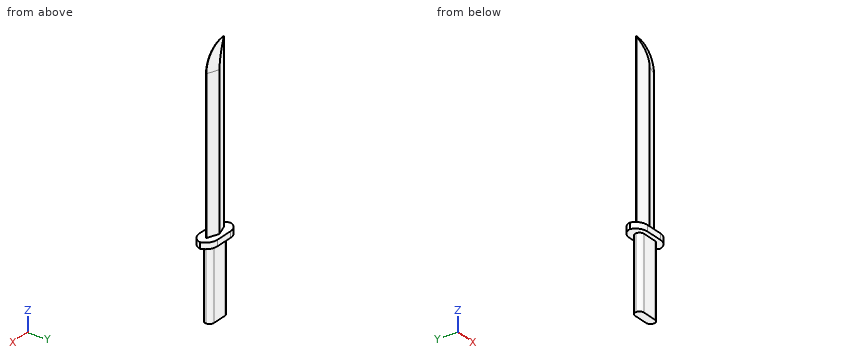
from build123d import *

# Parameters (mm, degrees)
F1_DEPTH     = 19.05
F2_W         = 88.9
F2_H         = 38.1
F3_DEPTH     = 12.7
F4_W         = 50.8
F4_H         = 381
F5_DEPTH     = 19.05
F6_R         = 50.79999
F7_T1_DEPTH  = 434.1925462068
F7_T3_DEPTH  = 317.50001
F7_T5_DEPTH  = 65.8925562068
F7_T8_ANGLE  = 90
F7_T10_ANGLE = 90
F8_R         = 9.52499
F9_T1_DEPTH  = 139.7


# Not quite as in the source:
# - a fillet or chamfer that OpenCascade refuses, or shapes differently, is made with other operations: its cross-section is extruded or revolved along the edge and cut away or added
# - a fillet or chamfer is up to 0.001 mm smaller than in the source, because OpenCascade refuses the exact size


with BuildPart() as f1:
    # F0 (on Front) → F1 (new body)
    with BuildSketch(Plane.XZ):
        Polygon((-25.4, -86.237093463), (0, -86.237093463), (25.4, -86.237093463), (25.4, 66.162906537), (-25.4, 66.162906537), align=None)
    extrude(amount=F1_DEPTH)

    # F2 (on face) → F3 (join)
    with BuildSketch(Plane.XY.offset(66.162906537)):
        with Locations((0, -9.525)):
            Rectangle(F2_W, F2_H)
    extrude(amount=F3_DEPTH)

    # F4 (on face) → F5 (join)
    with BuildSketch(Plane(origin=(0, 0, 0), x_dir=(-1, 0, 0), z_dir=(0, 1, 0))):
        with Locations((0, 256.662906537)):
            Rectangle(F4_W, F4_H)
    extrude(amount=-F5_DEPTH)

    # F6 (radius 50.8 in the source; OpenCascade refuses exactly that, so slightly less here)
    f6_edges = [f1.edges().sort_by_distance(p)[0] for p in [
        (25.4, -9.525, 447.162907),
    ]]
    fillet(f6_edges, radius=F6_R)

    # F7: chamfer of 25.4 x 9.2448439504 on 6 edges, made by hand

    # F7_s2 → F7_t1 (cut)
    with BuildSketch(Plane.XY.offset(78.862906537)):
        Polygon((0, 0), (-25.4, -9.2448439504), (-25.4, 0), align=None)
        Polygon((0, -19.05), (-25.4, -9.8051560496), (-25.4, -19.05), align=None)
    extrude(amount=F7_T1_DEPTH, mode=Mode.SUBTRACT)

    # F7_s4 → F7_t3 (cut)
    with BuildSketch(Plane.XY.offset(78.862906537)):
        Polygon((25.4, -9.2448439504), (0, 0), (25.4, 0), align=None)
        Polygon((25.4, -9.8051560496), (0, -19.05), (25.4, -19.05), align=None)
    extrude(amount=F7_T3_DEPTH, mode=Mode.SUBTRACT)

    # F7_s6 → F7_t5 (cut)
    with BuildSketch(Plane.YZ.offset(-91.2925462068)):
        Polygon((-19.05, 421.762906537), (-9.8051560496, 447.162906537), (-19.05, 447.162906537), align=None)
        Polygon((0, 421.762906537), (-9.2448439504, 447.162906537), (0, 447.162906537), align=None)
    extrude(amount=F7_T5_DEPTH, mode=Mode.SUBTRACT)

    # F7_s7 → F7_t8 (revolve, cut)
    with BuildSketch(Plane.XY.offset(396.362916537)):
        Polygon((0, 0), (25.4, -9.2448439504), (25.4, 0), align=None)
    revolve(axis=Axis((-25.39999, 0, 396.362916537), (0, -1, 0)), revolution_arc=F7_T8_ANGLE, mode=Mode.SUBTRACT)

    # F7_s9 → F7_t10 (revolve, cut)
    with BuildSketch(Plane.XY.offset(396.362916537)):
        Polygon((25.4, -9.8051560496), (0, -19.05), (25.4, -19.05), align=None)
    revolve(axis=Axis((-25.39999, -19.05, 396.362916537), (0, -1, 0)), revolution_arc=F7_T10_ANGLE, mode=Mode.SUBTRACT)

    # F8 (radius 9.525 in the source; OpenCascade refuses exactly that, so slightly less here)
    f8_edges = [f1.edges().sort_by_distance(p)[0] for p in [
        (25.4, 0, -10.037093),
        (-25.4, 0, -10.037093),
        (-25.4, -19.05, -10.037093),
        (25.4, -19.05, -10.037093),
    ]]
    fillet(f8_edges, radius=F8_R)

    # F9: fillet of radius 25.4 on 4 edges, made by hand

    # F9_s2 → F9_t1 (cut)
    with BuildSketch(Plane.XY.offset(2.662906537)):
        with BuildLine():
            ThreePointArc((19.05, -28.575), (37.0105122421, -21.1355122421), (44.45, -3.175))
            Line((44.45, -3.175), (44.45, -28.575))
            Line((44.45, -28.575), (19.05, -28.575))
        make_face()
        with BuildLine():
            ThreePointArc((19.05, 9.525), (37.0105122421, 2.0855122421), (44.45, -15.875))
            Line((44.45, -15.875), (44.45, 9.525))
            Line((44.45, 9.525), (19.05, 9.525))
        make_face()
        with BuildLine():
            ThreePointArc((-44.45, -3.175), (-37.0105122421, -21.1355122421), (-19.05, -28.575))
            Line((-19.05, -28.575), (-44.45, -28.575))
            Line((-44.45, -28.575), (-44.45, -3.175))
        make_face()
        with BuildLine():
            ThreePointArc((-44.45, -15.875), (-37.0105122421, 2.0855122421), (-19.05, 9.525))
            Line((-19.05, 9.525), (-44.45, 9.525))
            Line((-44.45, 9.525), (-44.45, -15.875))
        make_face()
    extrude(amount=F9_T1_DEPTH, mode=Mode.SUBTRACT)


solid = f1.part
Input: part model. Units: mm. Frame: model coordinates. Round coordinates to 2 decimals unless told otherwise and drop trailing zeros. Loops run counter-clockwise (first coordinate to the right, second up) from the corner with the lowest first, then second, coordinate; pieces in that order, holes last. Notation, with made-up numbers: (79.5, 11) -> (138.5, 11) arc R16 cw to (138.5, 29) -> close; hole circle Ø4 at (-24, 74). An arc over 180 degrees is marked (long way). Answer as a JSON object with one key per item and string values. Group by question number.
1) Section query A-A on z = 86. Output: boundary loops of the cut face in (x, y), plus the area to 3 significant figures.
2) Section query D-D on x = -35. Output: boundary loops of the cut face in (y, z).
3) Section query B-B on x = 31. Output: boundary loops of the cut face in (y, z), plus the area to 3 significant figures.
4) Ray query, L1, parallel to Z at x = -30.5, y = -12.5; L2, parallel to Y at x = 17, z = -63; L3, parallel to Y at x = -3, z = 3.5. Return the intervals inside material, ascending.
5) Pin query (flat end, axial travel): pin 1 (3 mm diameter, centred on x = -12, z = 386, fed in from +Y); pin 2 (2 mm diameter, centred on x = -14.5, y = -1.5, fed in from +Z); pin 3 (6 mm diameter, centred on y = 5.5, z = 240.5, fed in from -X); pin 4 (0.6 mm diameter, centred on y = -9.5, z = 188.5, fed in from +X). Return the tip coordinate at first contact, or that it passes through.
Reply:
{
 "1": {"outline": "(-25.4, -9.81) -> (0, -19.05) -> (25.4, -9.81) -> (25.4, -9.24) -> (0, 0) -> (-25.4, -9.24) -> close", "area": "498 mm2"},
 "2": {"outline": "(-22.94, 66.16) -> (3.89, 66.16) -> (3.89, 78.86) -> (-22.94, 78.86) -> close"},
 "3": {"outline": "(-25.59, 66.16) -> (6.54, 66.16) -> (6.54, 78.86) -> (-25.59, 78.86) -> close", "area": "408 mm2"},
 "4": {"L1": "z = 66.16 to 78.86", "L2": "y = -18.98 to -0.07", "L3": "y = -19.05 to 0"},
 "5": {"pin 1": "stops at y = -3.82", "pin 2": "stops at z = 78.86", "pin 3": "passes through", "pin 4": "stops at x = 25.4"}
}
